Verification items for this drawing (mm, ordinates from the low corner). A direction names the side the tool comes from. Round coordinates to 2 decimals unless told otherwise and drop trailing zeros. Order: outer loops, then holes, each group sorted by start corner. A loop starts at its lowest first (then second) coordinate and runs counter-clockwise, first axis right, second up. Notation, with made-up numbers: (83, -26) - (100, -26) arc R17 ccw to (100, -16) - close; hole circle Ø5 at (-3.5, -34). An arc over 180 degrees is marked (long way). One line per question, with ' | ' between items. Start each with the question number.
Q1. Material ranges on line 1 along Y through (x, z) = (6, 6); line 2 along Y through (x, z) = (6, 63); line 3 along Z through (x, y) = (8.5, 2), recorded low to high.
Q2. Gauge pin test, flat ends, axial feed: P1, Ø0.8, axis at x = 6.5, y = 6, coming from the -Z side; P2, Ø1, axis at y = 6, z = 16, coming from the -X side; P3, Ø2, axis at y = 9, z = 29, coming from the -X side. Record the tip position at first contact, or that the pin passes through.
Q3. Tool access check on the marked faces 1 and 2. Record the directions out of +Z, -Z, +X, -X, +Y, -Y that give a thin tool (end or side, any length) a straight path to the whole face; none if there is none.
Q4. Sectioned sample at A-A, the plane x = 6. Enter the section's corners in (y, z).
Q5. Sectioned sample at C-C, the plane y = 3.5. Enter the section's corners in (x, z).
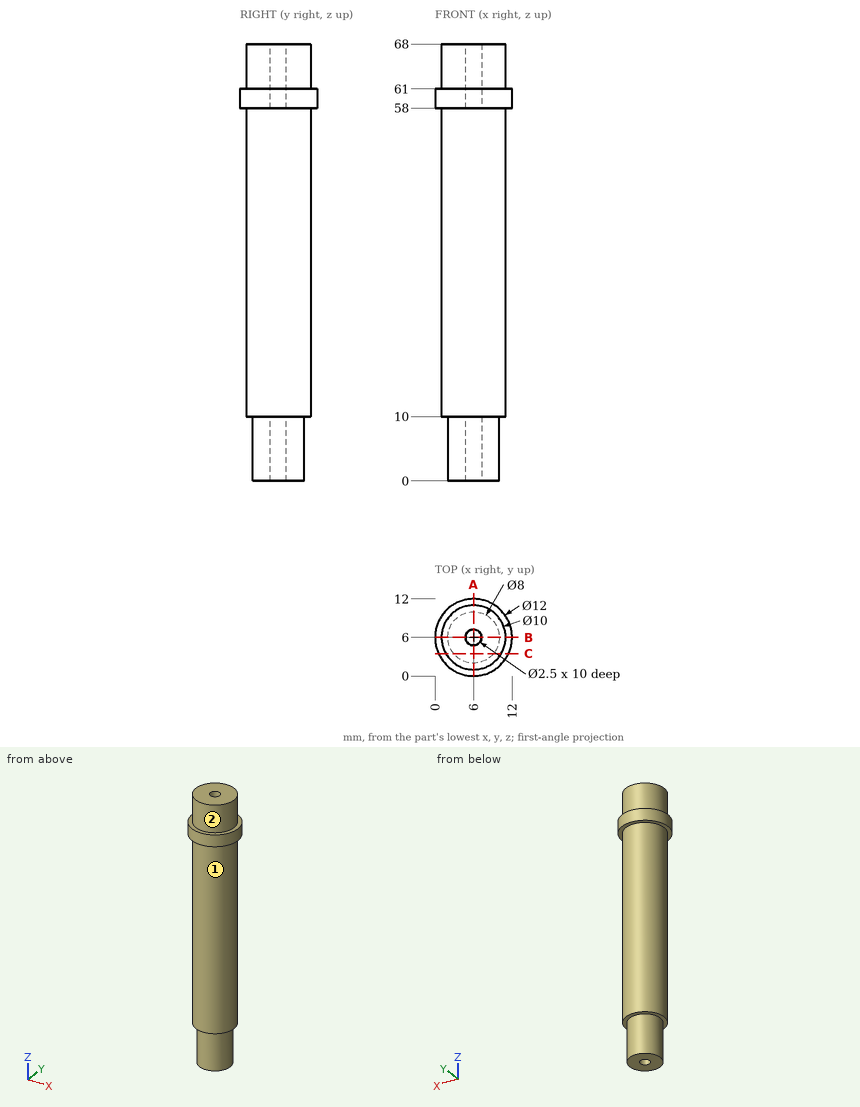
Determined:
1) line 1: y = 2 to 4.75, 7.25 to 10 | line 2: y = 1 to 4.75, 7.25 to 11 | line 3: z = 10 to 68
2) P1: stops at z = 10 | P2: stops at x = 1 | P3: stops at x = 1.42
3) face 1: -Z | face 2: +Z
4) outline: (0, 58) - (1, 58) - (1, 10) - (2, 10) - (2, 0) - (4.75, 0) - (4.75, 10) - (7.25, 10) - (7.25, 0) - (10, 0) - (10, 10) - (11, 10) - (11, 58) - (12, 58) - (12, 61) - (11, 61) - (11, 68) - (7.25, 68) - (7.25, 58) - (4.75, 58) - (4.75, 68) - (1, 68) - (1, 61) - (0, 61) - close
5) outline: (0.55, 58) - (1.67, 58) - (1.67, 10) - (2.88, 10) - (2.88, 0) - (9.12, 0) - (9.12, 10) - (10.33, 10) - (10.33, 58) - (11.45, 58) - (11.45, 61) - (10.33, 61) - (10.33, 68) - (1.67, 68) - (1.67, 61) - (0.55, 61) - close
